from build123d import *

# Parameters (mm, degrees)
F0_W     = 1100
F0_H     = 600
F1_DEPTH = 20
F2_W     = 50
F2_H     = 25
F2_W_2   = 25
F3_DEPTH = 20.001
F5_D     = 5
F6_SIZE  = 5


with BuildPart() as f1:
    # F0 (on Top) → F1 (new body)
    with BuildSketch(Plane.XY):
        Rectangle(F0_W, F0_H)
    extrude(amount=F1_DEPTH)

    # F2 (on face) → F3 (cut, through all)
    with BuildSketch(Plane.XY.offset(20)):
        with BuildLine():
            Line((473.75, -216.25), (473.75, -123.75))
            ThreePointArc((473.75, -123.75), (472.65165, -121.09835), (470, -120))
            ThreePointArc((470, -120), (467.34835, -121.09835), (466.25, -123.75))
            Line((466.25, -123.75), (466.25, -216.25))
            ThreePointArc((466.25, -216.25), (467.34835, -218.90165), (470, -220))
            ThreePointArc((470, -220), (472.65165, -218.90165), (473.75, -216.25))
        make_face()
        with BuildLine():
            Line((473.75, -46.25), (473.75, 46.25))
            ThreePointArc((473.75, 46.25), (472.65165, 48.90165), (470, 50))
            ThreePointArc((470, 50), (467.34835, 48.90165), (466.25, 46.25))
            Line((466.25, 46.25), (466.25, -46.25))
            ThreePointArc((466.25, -46.25), (467.34835, -48.90165), (470, -50))
            ThreePointArc((470, -50), (472.65165, -48.90165), (473.75, -46.25))
        make_face()
        with BuildLine():
            Line((466.25, 216.25), (466.25, 123.75))
            ThreePointArc((466.25, 123.75), (467.34835, 121.09835), (470, 120))
            ThreePointArc((470, 120), (472.65165, 121.09835), (473.75, 123.75))
            Line((473.75, 123.75), (473.75, 216.25))
            ThreePointArc((473.75, 216.25), (472.65165, 218.90165), (470, 220))
            ThreePointArc((470, 220), (467.34835, 218.90165), (466.25, 216.25))
        make_face()
        with Locations((-550, 0)):
            Rectangle(F2_W, F2_H)
        with Locations((550, 0)):
            Rectangle(F2_W, F2_H)
        with Locations((-537.5, 287.5)):
            Rectangle(F2_W_2, F2_H)
        with Locations((537.5, 287.5)):
            Rectangle(F2_W_2, F2_H)
    extrude(amount=-F3_DEPTH, mode=Mode.SUBTRACT)

    # F5 (through all)
    with Locations(Plane.XY.offset(20)):
        with Locations((537.5, -287.5), (-537.5, -287.5), (537.5, 262.5), (-537.5, 262.5)):
            Hole(F5_D / 2)

    # F6
    f6_edges = [f1.edges().sort_by_distance(p)[0] for p in [
        (0, -300, 20),
        (-550, -156.25, 20),
        (-550, 143.75, 20),
        (0, 300, 20),
        (550, -156.25, 20),
        (550, 143.75, 20),
    ]]
    chamfer(f6_edges, length=F6_SIZE)


solid = f1.part
Input: part model. Units: mm. Frame: model coordinates. A direction names the side the tool comes from. Give positions to 0.01 mm unless a question says otherwise; leave off trailing zeros. Use CSV: the item, a comma, the result in double quotes. Start each with the question number.
Item 1: Mould query, pull axis X, two halves, no side actions, for faces 1 (the flat face through (473.75, 169, 10)), 2 (the flat face through (-525, 0, 10)), 3 (the flat face through (-538, 12.5, 10)). Classes: pulls with the +X half, pulls with the -X half, needs draft (parallel to the pull), parting line crosses it, or undercut.
Item 2: Contact query for flat-ended pins moving along their axis: P1, Ø10, axis at x = 20, y = -149, coming from the -Z side; P2, Ø6, axis at y = -1.5, z = 9, coming from the +X side; P3, Ø1.5, axis at x = -22.5, z = 17.5, coming from the +Y side; P4, Ø6, axis at x = -543, z = 12.5, coming from the +Y side. Output: stop coordinate, or through.
Item 3: Reachability of faces 4 (the flat face through (-538, -12.5, 10)), 5 (the flat face through (537, 275, 10)), 6 (the flat face through (537, 12.5, 10)), 7 (the flat face through (466.25, 1, 10)) from +Z, -Z, +X, -X, +Y, -Y: full face, straight path, thin tool, end or side. Return the list, or none.
Item 4: Line query: line 1 (Y direction, x = -537.5, z = 15.25); line 2 (Y direction, x = -537.5, z = 10.25); line 3 (X direction, y = -287.5, z = 13.5). Output: solid intervals per line, ascending.
Ans:
1,face 1,"undercut"
1,face 2,"pulls with the -X half"
1,face 3,"needs draft"
2,P1,"stops at z = 0"
2,P2,"stops at x = 525"
2,P3,"stops at y = 298.25"
2,P4,"stops at y = 275"
3,face 4,"+Z, -Z, -X"
3,face 5,"+Z, -Z, +X, +Y"
3,face 6,"+Z, -Z, +X"
3,face 7,"+Z, -Z"
4,line 1,"y = -299.75 to -290, -285 to -12.5, 12.5 to 260, 265 to 275"
4,line 2,"y = -300 to -290, -285 to -12.5, 12.5 to 260, 265 to 275"
4,line 3,"x = -550 to -540, -535 to 535, 540 to 550"
